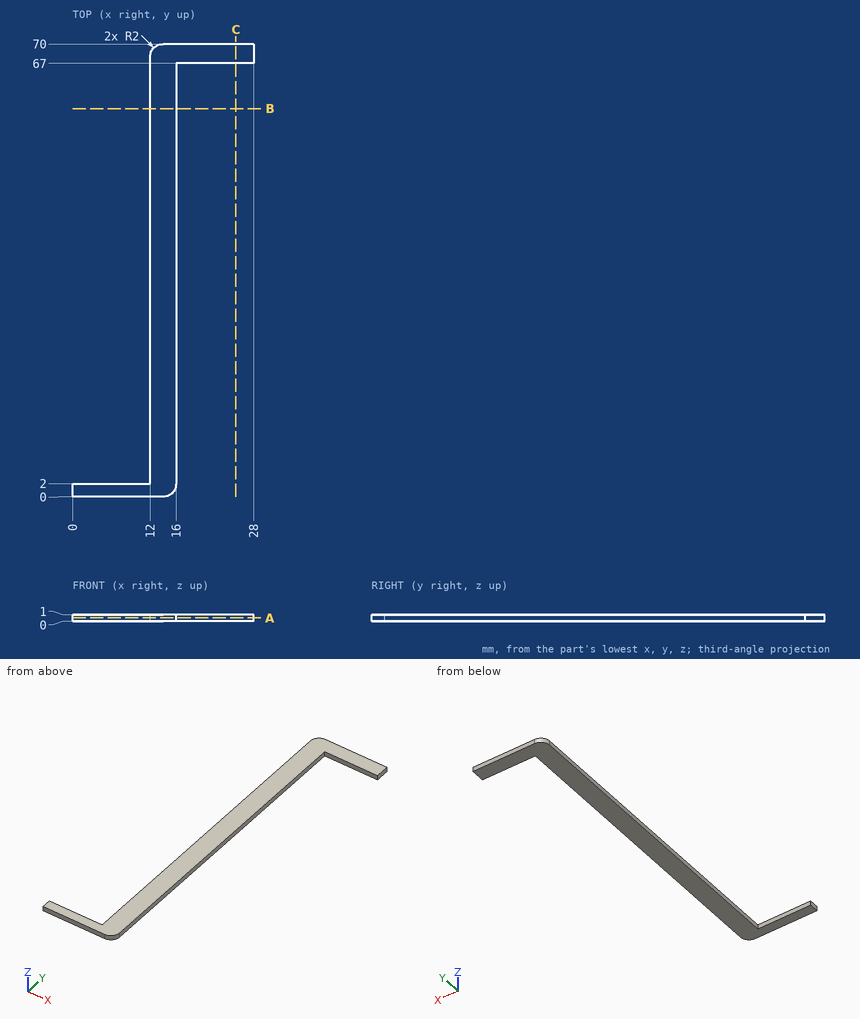
Input: dimensioned drawing with shaded views. Units: mm. Origin: part minimum x, y, z. Coordinates: 2 decimals unless noted, no trailing zeros. Order: outer loops, then holes, each group sorted by start corner. A loop starts at its lowest first (then second) coordinate and runs counter-clockwise, first axis right, second up. Notation, with made-up numbers: (-2, 20) - (53, 20) arc R15 ccw to (53, 44) - close; hole circle Ø10 at (84.25, -39). An arc over 180 degrees is marked (long way). Return JSON: item names as keys, results as strings. Group by question number.
1. Pin query (flat end, axial travel): pin 1 (0.5 mm diameter, centred on y = 46, z = 0.5, fed in from +X); pin 2 (0.5 mm diameter, centred on y = 28, z = 0.5, fed in from -X). Return the tip coordinate at first contact, or that it passes through.
2. Cut plane A-A (z = 0.55). Output: boundary loops of the cut face in (x, y).
3. Cut plane C-C (x = 25.25). Output: boundary loops of the cut face in (y, z), plus the area to 3 significant figures.
4. Cut plane B-B (y = 60). Output: boundary loops of the cut face in (x, z).
5. Material intervals for line 1 along Y through (x, z) = (21.5, 0.5); line 2 along X through (y, z) = (24.5, 0.9); line 3 along Y through (x, z) = (5, 0.25), sorted ascending. Write a range as [from, to].
Resolved:
{
 "1": {"pin 1": "stops at x = 16", "pin 2": "stops at x = 12"},
 "2": {"outline": "(0, 0) - (14, 0) arc R2 ccw to (16, 2) - (16, 67) - (28, 67) - (28, 70) - (14, 70) arc R2 ccw to (12, 68) - (12, 2) - (0, 2) - close"},
 "3": {"outline": "(67, 0) - (70, 0) - (70, 1) - (67, 1) - close", "area": "3.00 mm²"},
 "4": {"outline": "(12, 0) - (16, 0) - (16, 1) - (12, 1) - close"},
 "5": {"line 1": "y = [67, 70]", "line 2": "x = [12, 16]", "line 3": "y = [0, 2]"}
}
